Work out the finished part from the listing and answer in its coordinate system (mm). A direction names the side the tool comes from. Coordinates: 2 decimals unless noted, no trailing zeros. Order: outer loops, then holes, each group sorted by start corner. A loop starts at its lowest first (then second) coordinate and runs counter-clockwise, first axis right, second up. Notation, with made-up numbers: M 55,-8 L 92,-8 A12 ccw 92,11 Z; hole C -3,-36 d3. An arc over 180 degrees is marked long. Use a Markdown table: item, result.
from build123d import *

# Parameters (mm, degrees)
SKETCH1_R           = 27.5
SKETCH1_W           = 50.8
SKETCH1_H           = 50.8
BOSS_EXTRUDE1_DEPTH = 12.7
BOSS_EXTRUDE2_START = -3.175
SKETCH2_R           = 2
SKETCH2_W           = 50.8
SKETCH2_H           = 50.8
BOSS_EXTRUDE2_DEPTH = 3.175
SKETCH7_R           = 2
CUT_EXTRUDE4_DEPTH  = 10
SKETCH8_W           = 25.4
SKETCH8_H           = 75
CUT_EXTRUDE5_DEPTH  = 9.525


with BuildPart() as part:
    # Sketch1 → Boss-Extrude1 (new body)
    with BuildSketch(Plane.XY):
        with BuildLine():
            Line((30.675000233, 57.5), (30.675000233, -57.5))
            ThreePointArc((30.675000233, -57.5), (0, -88.175000233), (-30.675000233, -57.5))
            Line((-30.675000233, -57.5), (-30.675000233, 57.5))
            ThreePointArc((-30.675000233, 57.5), (0, 88.175000233), (30.675000233, 57.5))
        make_face()
        with Locations((0, -57.5)):
            Circle(SKETCH1_R, mode=Mode.SUBTRACT)
        with Locations(Location((0, 57.5, 0), (0, 0, 180))):
            Circle(SKETCH1_R, mode=Mode.SUBTRACT)
        Rectangle(SKETCH1_W, SKETCH1_H, mode=Mode.SUBTRACT)
    extrude(amount=BOSS_EXTRUDE1_DEPTH)

    # Sketch2 → Boss-Extrude2 (add)
    with BuildSketch(Plane.XY.offset(12.7).offset(BOSS_EXTRUDE2_START)):
        with BuildLine():
            Line((30.675000233, -57.5), (30.675000233, 57.5))
            ThreePointArc((30.675000233, 57.5), (0, 88.175000233), (-30.675000233, 57.5))
            Line((-30.675000233, 57.5), (-30.675000233, -57.5))
            ThreePointArc((-30.675000233, -57.5), (0, -88.175000233), (30.675000233, -57.5))
        make_face()
        with Locations((-1.290716795, 81.465267579)):
            Circle(SKETCH2_R, mode=Mode.SUBTRACT)
        with Locations((20.109172135, 70.600427323)):
            Circle(SKETCH2_R, mode=Mode.SUBTRACT)
        with Locations((21.39988893, 46.635159744)):
            Circle(SKETCH2_R, mode=Mode.SUBTRACT)
        with Locations((1.290716795, 33.534732421)):
            Circle(SKETCH2_R, mode=Mode.SUBTRACT)
        with Locations((-20.109172135, 44.399572677)):
            Circle(SKETCH2_R, mode=Mode.SUBTRACT)
        with Locations((-21.39988893, 68.364840256)):
            Circle(SKETCH2_R, mode=Mode.SUBTRACT)
        with Locations(Location((-21.39988893, -68.364840256, 0), (0, 0, 180))):
            Circle(SKETCH2_R, mode=Mode.SUBTRACT)
        with Locations(Location((-20.109172135, -44.399572677, 0), (0, 0, 180))):
            Circle(SKETCH2_R, mode=Mode.SUBTRACT)
        with Locations(Location((1.290716795, -33.534732421, 0), (0, 0, 180))):
            Circle(SKETCH2_R, mode=Mode.SUBTRACT)
        with Locations(Location((21.39988893, -46.635159744, 0), (0, 0, 180))):
            Circle(SKETCH2_R, mode=Mode.SUBTRACT)
        with Locations(Location((20.109172135, -70.600427323, 0), (0, 0, 180))):
            Circle(SKETCH2_R, mode=Mode.SUBTRACT)
        with Locations(Location((-1.290716795, -81.465267579, 0), (0, 0, 180))):
            Circle(SKETCH2_R, mode=Mode.SUBTRACT)
        Rectangle(SKETCH2_W, SKETCH2_H, mode=Mode.SUBTRACT)
    extrude(amount=BOSS_EXTRUDE2_DEPTH)

    # Sketch7 → Cut-Extrude4 (cut)
    with BuildSketch(Plane.ZY.offset(30.675000233)):
        with Locations(Location((4.7625, 0, 0), (0, 0, 270))):
            Circle(SKETCH7_R)
    cut_extrude4 = extrude(amount=-CUT_EXTRUDE4_DEPTH, mode=Mode.SUBTRACT)

    # Mirror2: Cut-Extrude4 across plane
    add(cut_extrude4.mirror(Plane(origin=(0, 0, 0), x_dir=(0, 0, 1), z_dir=(1, 0, 0))), mode=Mode.SUBTRACT)

    # Sketch8 → Cut-Extrude5 (cut)
    with BuildSketch(Plane(origin=(0, 0, 0), x_dir=(-1, 0, 0), z_dir=(0, 0, -1))):
        Rectangle(SKETCH8_W, SKETCH8_H)
    extrude(amount=-CUT_EXTRUDE5_DEPTH, mode=Mode.SUBTRACT)


solid = part.part
(1) A cutting plane is placed at A-A (y = 0). Determine the outline of the cut face in (x, z) (1 decimal).
Conclusion:
| item | result |
|---|---|
| outline | M -30.7,0 L -25.4,0 L -25.4,2.8 L -30.7,2.8 Z; M -30.7,6.8 L -25.4,6.8 L -25.4,12.7 L -30.7,12.7 Z; M 25.4,0 L 30.7,0 L 30.7,2.8 L 25.4,2.8 Z; M 25.4,6.8 L 30.7,6.8 L 30.7,12.7 L 25.4,12.7 Z |
(2) Given P1, Ø4.5, axis at x = 21.4, y = -46.64, coming from the -Z side (3 decimals); P2, Ø6, axis at x = 12.5, z = 2, coming from the +Y side; P3, Ø6.5, axis at x = 0.5, z = 6, coming from the +Y side (3 decimals), each flat-ended and moving along its own axis, determine where each tip first touches the part or whether it passes through.
Conclusion:
| item | result |
|---|---|
| P1 | z = 9.525 |
| P2 | y = 86.67 |
| P3 | y = 88.175 |
(3) Determine the mould class of faces 1 (the cylindrical face through (21.66, -48.62, 11.09)), 2 (the flat face through (-27, 1, 12.7)) for opening direction Y: pulls with the +Y half, pulls with the -Y half, needs draft (parallel to the pull), parting line crosses it, or undercut.
Conclusion:
| item | result |
|---|---|
| face 1 | undercut |
| face 2 | needs draft |
(4) Which of the six approach directions +Z, -Z, +X, -X, +Y, -Y give full straight-line access (tool end or side, diameter ignored) to faces 3 (the cylindrical face through (28.074, 0.26, 6.745)), 4 (the flat face through (0, 25.4, 10)), 5 (the cylindrical face through (-1.02, -84.98, 4.7))?
Conclusion:
| item | result |
|---|---|
| face 3 | +X, -X |
| face 4 | +Z, -Z |
| face 5 | -Z |
(5) Straight lines are drawn through the part: L1, parallel to Y at x = 1.5, z = 11.75; L2, parallel to Y at x = -22.5, z = 3.5; L3, parallel to X at y = 1.5, z = 11.5 (3 decimals). For each, find the intervals that lie inside material, in ascending order.
Conclusion:
| item | result |
|---|---|
| L1 | -88.14 to -35.52, -31.55 to -25.4, 25.4 to 31.55, 35.52 to 88.14 |
| L2 | -78.35 to -73.31, -41.69 to -25.4, 25.4 to 41.69, 73.31 to 78.35 |
| L3 | -30.675 to -25.4, 25.4 to 30.675 |
(6) A cutting plane is placed at B-B (x = -11). Determine the outline of the cut face in (y, z) (3 decimals), then the cut area to 3 significant figures.
Conclusion:
| item | result |
|---|---|
| outline | M -86.135,0 L -82.704,0 L -82.704,9.525 L -25.4,9.525 L -25.4,12.7 L -86.135,12.7 Z; M 25.4,9.525 L 82.704,9.525 L 82.704,0 L 86.135,0 L 86.135,12.7 L 25.4,12.7 Z |
| area | 451 mm2 |
